```python
from build123d import *

# Parameters (mm, degrees)
SKETCH1_W           = 84
SKETCH1_H           = 62
BOSS_EXTRUDE1_DEPTH = 4
CUT_EXTRUDE2_DEPTH  = 5


with BuildPart() as part:
    # Sketch1 → Boss-Extrude1 (new body)
    with BuildSketch(Plane.XY):
        with Locations((0.5, 0)):
            Rectangle(SKETCH1_W, SKETCH1_H)
    extrude(amount=BOSS_EXTRUDE1_DEPTH)

    # Sketch3 → Cut-Extrude2 (cut)
    with BuildSketch(Plane.XY.offset(4)):
        Polygon((-27.1, 22.6), (-27.1, 12.6), (-31.5, 12.6), (-31.5, 22.6), (-33, 22.6), (-33, 26), (-31.5, 26), (-31.5, 31), (-27.1, 31), (-27.1, 26), (-25.6, 26), (-25.6, 22.6), align=None)
        Polygon((31.5, 12.6), (31.5, 22.6), (33, 22.6), (33, 26), (31.5, 26), (31.5, 31), (27.1, 31), (27.1, 26), (25.6, 26), (25.6, 22.6), (27.1, 22.6), (27.1, 12.6), align=None)
        Polygon((-31.5, -12.6), (-31.5, -22.6), (-33, -22.6), (-33, -26), (-31.5, -26), (-31.5, -31), (-27.1, -31), (-27.1, -26), (-25.6, -26), (-25.6, -22.6), (-27.1, -22.6), (-27.1, -12.6), align=None)
    extrude(amount=-CUT_EXTRUDE2_DEPTH, mode=Mode.SUBTRACT)


solid = part.part
```
Verification items for the finished model (mm, model axes). A direction names the side the tool comes from. Give positions to 0.01 mm unless a question says otherwise; leave off trailing zeros. Order: outer loops, then holes, each group sorted by start corner. A loop starts at its lowest first (then second) coordinate and runs counter-clockwise, first axis right, second up. Notation, with made-up numbers: M 20.25,60.5 L 27.25,60.5 A22 ccw 27.25,75.5 Z; hole C 82,22.25 d6. An arc over 180 degrees is marked long. Return JSON: item names as keys, results as strings. Group by question number.
1) Section check A-A on y = 20.5. Record the cut outline in (x, z), and give its area (3 significant figures).
2) Scan lines: line 1 (X direction, y = 19, z = 3.2); line 2 (X direction, y = -14, z = 2.4); line 3 (Y direction, x = 30, z = 0.65). Record each from-to range of solid material in increasing order.
3) Mould release check, pull along Y, two halves, no side actions. Record for faces 1 (the face through (-37, -31, 2)), 2 (the face through (-33, -24, 2)), 3 (the face through (-31.5, 28, 2)), 4 (the face through (-37, 31, 2)): pulls with the +Y half, pulls with the -Y half, needs draft (parallel to the pull), parting line crosses it, or undercut.
4) Access from +Z, -Z, +X, -X, +Y, -Y to the whole of each face (thin tool, end or side, straight path). Record for faces 5 (the face through (-25.6, 24, 2)), 6 (the face through (-27.1, -18, 2)), 7 (the face through (37, 31, 2)), 8 (the face through (0, 0, 0)), 9 (the face through (31.5, 18, 2)).
Answer block:
{
 "1": {"outline": "M -41.5,0 L -31.5,0 L -31.5,4 L -41.5,4 Z; M -27.1,0 L 27.1,0 L 27.1,4 L -27.1,4 Z; M 31.5,0 L 42.5,0 L 42.5,4 L 31.5,4 Z", "area": "301 mm^2"},
 "2": {"line 1": "x = -41.5 to -31.5, -27.1 to 27.1, 31.5 to 42.5", "line 2": "x = -41.5 to -31.5, -27.1 to 42.5", "line 3": "y = -31 to 12.6"},
 "3": {"face 1": "pulls with the -Y half", "face 2": "undercut", "face 3": "needs draft", "face 4": "pulls with the +Y half"},
 "4": {"face 5": "+Z, -Z", "face 6": "+Z, -Z, -Y", "face 7": "+Z, -Z, +X, -X, +Y", "face 8": "-Z, +X, -X, +Y, -Y", "face 9": "+Z, -Z, +Y"}
}
